For this review, take the finished solid that the model builds, in its own axes (mm). A direction names the side the tool comes from. Coordinates: 2 decimals unless noted, no trailing zeros. Write each loop counter-clockwise with the first axis right and the second up, starting at its lowest first coordinate (ties: lowest second). Pieces come first, ordered by that corner, then holes. Notation, with made-up numbers: (49.25, 41.5) -> (89.25, 41.5) arc R13 cw to (89.25, 66.5) -> close; hole circle Ø5 at (88, 50). An arc over 180 degrees is marked (long way). Put each result on its own line as item: value. Start each with the question number.
Item 1: Consider section A-A on x = 22.25. Give the boundary of the cut face in (y, z).
Item 2: The part is to be moulded in two halves that separate along X. For faces 1 (the flat face through (20, 7.75, 3)), 2 (the cylindrical face through (-25.965, -10.199, 0.76)), 3 (the flat face through (0, -7.75, 3)), say which applies: +X half, -X half, draft (parallel to the pull), parting line (faces both ways), or undercut.
Item 3: Insertion check: P1, Ø2, axis at y = 4.5, z = 4, coming from the +X side; P2, Ø3, axis at x = -2.5, z = 3.5, coming from the -Y side; P3, Ø1, axis at x = 18, z = 3, coming from the +Y side; P4, Ø5, axis at x = -20, y = -3, coming from the +Z side. Each pin has a flat end and moves straight along its axis. Give the tip position at first contact, or say it passes through.
Item 4: For faces 4 (the flat face through (-24.45, 6, 3)), 5 (the flat face through (20, -7.75, 3)), 6 (the cylindrical face through (-10.56, 8.82, 3.23)), 7 (the flat face through (17.5, 0, 3)), 8 (the cylindrical face through (-10.44, -8.82, 3.23)), list the 3-axis set-ups (+Z, -Z, +X, -X, +Y, -Y) from which the entire face can be reached by the end or side of a thin tool; tool diameter is ignored.
Item 5: Consider section B-B on y = -5.5. Give the boundary of the cut face in (x, z), and give its area (3 significant figures).
Item 6: To check wall thickness, follow L1, parallel to X at y = -5.5, z = 0.4; L2, parallel to Y at x = -22.25, z = 2.05; L3, parallel to X at y = 5.5, z = 2.65. State the ranges of each line that lie inside material, in increasing order.
Item 7: Consider section D-D on y = 5.5. Give the boundary of the cut face in (x, z).
Item 8: Consider section C-C on z = 3.6. Give the boundary of the cut face in (x, y), and give its area (3 significant figures).
Autodesk Inventor part; units mm, degrees
ref_plane "YZ Plane" through (0, 0, 0) normal (1, 0, 0) x (0, 1, 0)
ref_plane "XZ Plane" through (0, 0, 0) normal (0, 1, 0) x (-1, 0, 0)
ref_plane "XY Plane" through (0, 0, 0) normal (0, 0, 1) x (1, 0, 0)
sketch "スケッチ1" plane through (0, 0, 0) normal (0, 0, 1) x (1, 0, 0)
  line L0 (-26.25, 10.5) -> (26.25, 10.5)
  line L1 (26.25, 10.5) -> (26.25, -10.5)
  line L2 (26.25, -10.5) -> (-26.25, -10.5)
  line L3 (-26.25, -10.5) -> (-26.25, 10.5)
  point P0 (0, 0)
  dimension "d0" = 52.5
  dimension "d1" = 21
  dimension "d2" = 10.5
  dimension "d3" = 26.25
extrude "押し出し1" add sketch "スケッチ1" along normal blind 1.5
sketch "スケッチ6" plane through (0, 0, 1.5) normal (0, 0, 1) x (1, 0, 0)
  line L0 (-24.45, -7.75) -> (-24.45, 7.75)
  line L1 (24.45, 7.75) -> (24.45, -7.75)
  line L2 (24.45, -7.75) -> (14.6971, -7.75)
  arc A0 (14.7186, 7.75) -> (6.2813, 7.75) centre (10.5, -0.0198) ccw
  arc A1 (6.3028, -7.75) -> (14.6971, -7.75) centre (10.5, -0.0198) ccw
  line L3 (14.7186, 7.75) -> (24.45, 7.75)
  line L4 (6.3028, -7.75) -> (-6.2921, -7.75)
  line L5 (-14.7079, -7.75) -> (-24.45, -7.75)
  arc A2 (-6.2921, 7.75) -> (-14.7079, 7.75) centre (-10.5, 0) ccw
  arc A3 (-14.7079, -7.75) -> (-6.2921, -7.75) centre (-10.5, 0) ccw
  line L6 (-24.45, 7.75) -> (-14.7079, 7.75)
  line L7 (-6.2921, 7.75) -> (6.2813, 7.75)
  point P0 (0, 0)
  dimension "d86" = 48.9
  dimension "d87" = 15.5
  dimension "d89" = 24.45
  dimension "d92" = 10.5
  dimension "d93" = 10.5
  dimension "d97" = 15.5
  dimension "d98" = 7.75
  dimension "d99" = 7.75
  dimension "d100" = 7.75
  dimension "d101" = 7.75
  dimension "d102" = 7.75
  dimension "d103" = 57
  dimension "d104" = 57
  dimension "d105" = 57
  dimension "d106" = 57
extrude "押し出し4" add sketch "スケッチ6" along normal blind 3.5
sketch "スケッチ7" plane through (0, 0, 5) normal (0, 0, 1) x (1, 0, 0)
  point P0 (0, 0)
  point P1 (-22.25, 5.5)
  point P2 (-22.25, -5.5)
  point P3 (22.25, 5.5)
  point P4 (22.25, -5.5)
  dimension "d62" = 44.5
  dimension "d63" = 11
  dimension "d64" = 11
  dimension "d65" = 44.5
  dimension "d66" = 22.25
  dimension "d67" = 5.5
  dimension "d68" = 22.25
  dimension "d69" = 5.5
hole "穴3" at (-22.25, 5.5, 5) at (-22.25, -5.5, 5) at (22.25, 5.5, 5) at (22.25, -5.5, 5) direction (0, 0, -1) diameter 2.2 end through all
fillet "フィレット3" radius 1 4 edges at (-26.25, -10.5, 0.75) (26.25, -10.5, 0.75) (26.25, 10.5, 0.75) (-26.25, 10.5, 0.75)
sketch "スケッチ8" plane through (0, 0, 5) normal (0, 0, 1) x (1, 0, 0)
  line L0 (-10.5, -5) -> (17.5, -5)
  line L1 (17.5, -5) -> (17.5, 5)
  line L2 (17.5, 5) -> (-17.5, 5)
  line L3 (-24.45, 7.75) -> (-24.45, -7.75)
  line L4 (-20, -4) -> (-24.45, -4)
  line L5 (-24.45, -4) -> (-24.45, 4)
  line L6 (-24.45, 4) -> (-17.5, 4)
  line L7 (-25.25, -10.5) -> (25.25, -10.5)
  line L8 (25.25, 10.5) -> (-25.25, 10.5)
  line L9 (-17.5, 5) -> (-17.5, 4)
  line L10 (-10.5, -5) -> (-10.5, -6.5)
  line L11 (-10.5, -6.5) -> (-17.5, -6.5)
  line L12 (-17.5, -6.5) -> (-20, -6.5)
  line L13 (-20, -6.5) -> (-20, -4)
  point P0 (0, 0)
  dimension "d80" = 35
  dimension "d81" = 10
  dimension "d82" = 5
  dimension "d95" = 6.5
  dimension "d109" = 1.5
  dimension "d111" = 9.5
extrude "押し出し5" cut sketch "スケッチ8" against normal blind 3.55
equation "\"d102\" = 0.5 * d97"
equation "\"d95\" = d94"
equation "\"d20\" = 0.5 * d19"
equation "\"d44\" = 0.5 * d43"
equation "\"d55\" = 0.5 * d53"
equation "\"d83\" = 0.5 * d80"
equation "\"d88\" = 0.5 * d87"
properties part number "New_Accelite_Controller_Cover_copy_under" material "ABS プラスチック"
Return value:
1. outline: (-10.5, 0) -> (-6.6, 0) -> (-6.6, 5) -> (-7.75, 5) -> (-7.75, 1.5) -> (-10.5, 1.5) -> close; (-4.4, 0) -> (4.4, 0) -> (4.4, 5) -> (-4.4, 5) -> close; (6.6, 0) -> (10.5, 0) -> (10.5, 1.5) -> (7.75, 1.5) -> (7.75, 5) -> (6.6, 5) -> close
2. face 1: draft
2. face 2: -X half
2. face 3: undercut
3. P1: x = 24.45
3. P2: y = -7.75
3. P3: y = 7.75
3. P4: z = 5
4. face 4: +Z, -X, +Y, -Y
4. face 5: +Z, +X, -Y
4. face 6: +Z, +Y
4. face 7: +Z
4. face 8: +Z, -Y
5. outline: (-26.25, 0) -> (-23.35, 0) -> (-23.35, 5) -> (-24.45, 5) -> (-24.45, 1.5) -> (-26.25, 1.5) -> close; (-21.15, 0) -> (21.15, 0) -> (21.15, 5) -> (-10.5, 5) -> (-10.5, 1.45) -> (-20, 1.45) -> (-20, 5) -> (-21.15, 5) -> close; (23.35, 0) -> (26.25, 0) -> (26.25, 1.5) -> (24.45, 1.5) -> (24.45, 5) -> (23.35, 5) -> close
5. area: 194 mm^2
6. L1: -26.25 to -23.35, -21.15 to 21.15, 23.35 to 26.25
6. L2: -7.75 to -6.6, -4.4 to -4, 4 to 4.4, 6.6 to 7.75
6. L3: -24.45 to -23.35, -21.15 to 21.15, 23.35 to 24.45
7. outline: (-26.25, 0) -> (-23.35, 0) -> (-23.35, 5) -> (-24.45, 5) -> (-24.45, 1.5) -> (-26.25, 1.5) -> close; (-21.15, 0) -> (21.15, 0) -> (21.15, 5) -> (-21.15, 5) -> close; (23.35, 0) -> (26.25, 0) -> (26.25, 1.5) -> (24.45, 1.5) -> (24.45, 5) -> (23.35, 5) -> close
8. outline: (-24.45, -7.75) -> (-14.71, -7.75) arc R8.82 ccw to (-6.29, -7.75) -> (6.3, -7.75) arc R8.8 ccw to (14.7, -7.75) -> (24.45, -7.75) -> (24.45, 7.75) -> (14.72, 7.75) arc R8.84 ccw to (6.28, 7.75) -> (-6.29, 7.75) arc R8.82 ccw to (-14.71, 7.75) -> (-24.45, 7.75) -> (-24.45, 4) -> (-17.5, 4) -> (-17.5, 5) -> (17.5, 5) -> (17.5, -5) -> (-10.5, -5) -> (-10.5, -6.5) -> (-20, -6.5) -> (-20, -4) -> (-24.45, -4) -> close; hole circle Ø2.2 at (-22.25, -5.5); hole circle Ø2.2 at (-22.25, 5.5); hole circle Ø2.2 at (22.25, -5.5); hole circle Ø2.2 at (22.25, 5.5)
8. area: 345 mm^2
